Can you work these out from the drawing? Everything is in mm from the part's minimum corner. A direction names the side the tool comes from. Round coordinates to 2 decimals unless told otherwise and drop trailing zeros. One line per item, written item: value.
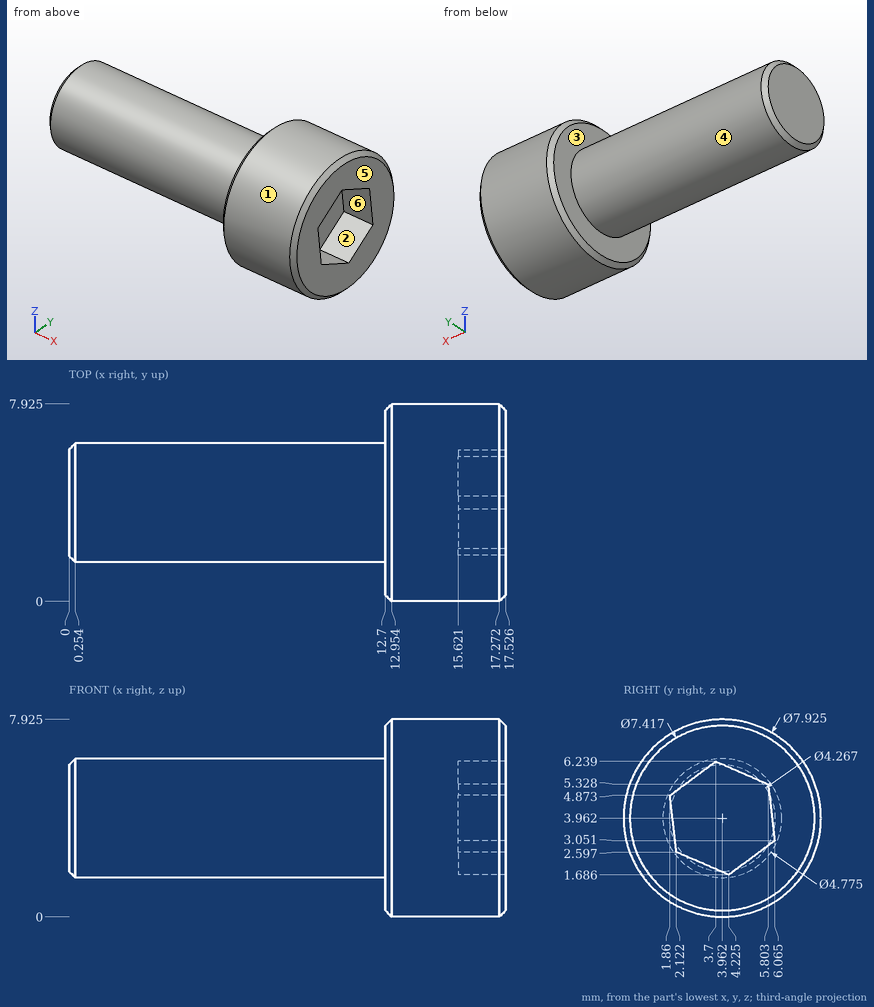
(1) We'd pull the mould along Y, two halves only. Please class the marked faces 4, 5 and 6: +Y half, -Y half, draft (parallel to the pull), parting line (faces both ways), or undercut.
Results below:
face 4: parting line
face 5: draft
face 6: undercut
(2) On a 3-axis mill with a long thin cutter (end or side, diameter ignored), from which of +Z, -Z, +X, -X, +Y, -Y can I reach the whole of each face in a straight line? I mean the marked faces 1, 2 and 3. Say none if no direction works.
Results below:
face 1: +X, -X
face 2: +X
face 3: -X
(3) Please list where these lines run through material, in increasing order: L1, parallel to X at y = 3.5, z = 0.5 (1 decimal); L2, parallel to X at y = 4.75, z = 2.25; L3, parallel to Z at x = 14, y = 6.5 (1 decimal).
Results below:
L1: x = 12.7 to 17.5
L2: x = 0 to 15.62
L3: z = 0.9 to 7
(4) For pin 1 Ø1 at (x, y) = (3, 5.5) entering from -Z; pin 2 Ø3 at (x, y) = (12, 1) entering from +Z; pin 3 Ø4 at (x, y) = (11, 6) entering from -Z, each with a flat end and sliding along its axis, tell me the tip position at first contact or that it passes through.
Results below:
pin 1: stops at z = 1.81
pin 2: stops at z = 7.49
pin 3: stops at z = 0.32
